from build123d import *

# Parameters (mm, degrees)
SKETCH1_R                    = 3.5
SKETCH1_R_2                  = 1.25
MOUNTING_BOSSES_DEPTH        = 4
MOUNTING_BOSSES_2_DEPTH      = 4
MOUNTING_BOSSES_3_DEPTH      = 4
MOUNTING_BOSSES_4_DEPTH      = 4
MATERIAL_BULK_DEPTH          = 33.5
SKETCH5_R                    = 1.25
MOUNT_POINT_CUT_REPEAT_DEPTH = 67
WEIGHT_RELIEF_DEPTH          = 67
FILLET2_R                    = 5
FILLET3_R                    = 10


with BuildPart() as part:
    # Sketch1 → MOUNTING BOSSES (new body)
    with BuildSketch(Plane.XY):
        with Locations((-30, 54.33)):
            Circle(SKETCH1_R)
        with Locations((-30, 54.33)):
            Circle(SKETCH1_R_2, mode=Mode.SUBTRACT)
    extrude(amount=MOUNTING_BOSSES_DEPTH)



with BuildPart() as body_2:
    # Sketch1 → MOUNTING BOSSES 2 (new body)
    with BuildSketch(Plane.XY):
        with Locations((30, 54.33)):
            Circle(SKETCH1_R)
        with Locations((30, 54.33)):
            Circle(SKETCH1_R_2, mode=Mode.SUBTRACT)
    extrude(amount=MOUNTING_BOSSES_2_DEPTH)


with BuildPart() as body_3:
    # Sketch1 → MOUNTING BOSSES 3 (new body)
    with BuildSketch(Plane.XY):
        with Locations((30, -54.33)):
            Circle(SKETCH1_R)
        with Locations((30, -54.33)):
            Circle(SKETCH1_R_2, mode=Mode.SUBTRACT)
    extrude(amount=MOUNTING_BOSSES_3_DEPTH)


with BuildPart() as body_4:
    # Sketch1 → MOUNTING BOSSES 4 (new body)
    with BuildSketch(Plane.XY):
        with Locations((-30, -54.33)):
            Circle(SKETCH1_R)
        with Locations((-30, -54.33)):
            Circle(SKETCH1_R_2, mode=Mode.SUBTRACT)
    extrude(amount=MOUNTING_BOSSES_4_DEPTH)


with BuildPart() as part_1:
    add(part.part)

    add(body_2.part)  # MATERIAL BULK merges body 2

    add(body_3.part)  # MATERIAL BULK merges body 3

    add(body_4.part)  # MATERIAL BULK merges body 4
    # Sketch4 → MATERIAL BULK (add, symmetric)
    with BuildSketch(Plane(origin=(0, 0, 0), x_dir=(0, 0, -1), z_dir=(1, 0, 0))):
        Polygon((-4, 54.33), (-4, 45.522585119), (0.5, 42.388948755), (0.5, -42.388948755), (-4, -45.522585119), (-4, -54.33), (0, -54.33), (0, -48.83), (5.5, -45), (5.5, 45), (0, 48.83), (0, 54.33), align=None)
    extrude(amount=MATERIAL_BULK_DEPTH, both=True)

    # Sketch5 → MOUNT POINT CUT REPEAT (cut)
    with BuildSketch(Plane.XY):
        with Locations((-30, 54.33)):
            Circle(SKETCH5_R)
        with Locations((30, 54.33)):
            Circle(SKETCH5_R)
        with Locations((30, -54.33)):
            Circle(SKETCH5_R)
        with Locations((-30, -54.33)):
            Circle(SKETCH5_R)
    extrude(amount=MOUNT_POINT_CUT_REPEAT_DEPTH, mode=Mode.SUBTRACT)

    # Sketch6 → WEIGHT RELIEF (cut)
    with BuildSketch(Plane.XY):
        with BuildLine():
            Line((-18.5, 30), (18.5, 30))
            ThreePointArc((18.5, 30), (22.035533906, 28.535533906), (23.5, 25))
            Line((23.5, 25), (23.5, 10))
            ThreePointArc((23.5, 10), (22.035533906, 6.464466094), (18.5, 5))
            Line((18.5, 5), (-18.5, 5))
            ThreePointArc((-18.5, 5), (-22.035533906, 6.464466094), (-23.5, 10))
            Line((-23.5, 10), (-23.5, 25))
            ThreePointArc((-23.5, 25), (-22.035533906, 28.535533906), (-18.5, 30))
        make_face()
        with BuildLine():
            Line((-18.5, -5), (18.5, -5))
            ThreePointArc((18.5, -5), (22.035533906, -6.464466094), (23.5, -10))
            Line((23.5, -10), (23.5, -25))
            ThreePointArc((23.5, -25), (22.035533906, -28.535533906), (18.5, -30))
            Line((18.5, -30), (-18.5, -30))
            ThreePointArc((-18.5, -30), (-22.035533906, -28.535533906), (-23.5, -25))
            Line((-23.5, -25), (-23.5, -10))
            ThreePointArc((-23.5, -10), (-22.035533906, -6.464466094), (-18.5, -5))
        make_face()
    extrude(amount=-WEIGHT_RELIEF_DEPTH, mode=Mode.SUBTRACT)

    # Fillet2
    fillet2_edges = [part_1.edges().sort_by_distance(p)[0] for p in [
        (0, 45.522585119, 4),
        (0, 42.388948755, -0.5),
        (0, -42.388948755, -0.5),
        (0, -45.522585119, 4),
        (0, -48.83, 0),
        (0, -45, -5.5),
        (0, 45, -5.5),
        (0, 48.83, 0),
    ]]
    fillet(fillet2_edges, radius=FILLET2_R)

    # Fillet3
    fillet3_edges = [part_1.edges().sort_by_distance(p)[0] for p in [
        (-26.5, 54.33, 2),
        (26.5, 54.33, 2),
        (26.5, -54.33, 2),
        (-26.5, -54.33, 2),
    ]]
    fillet(fillet3_edges, radius=FILLET3_R)


solid = part_1.part
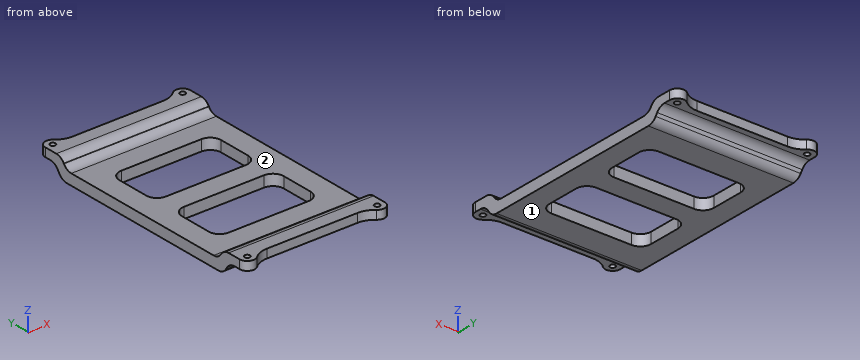
Geometry check sheet. Reference: the model listing, model coordinates, mm. Face numbers are marked on the shaded views. Give positions to 0.01 mm unless a question says otherwise; leave off trailing zeros. Write each loop counter-clockwise with the first axis right and the second up, starting at its lowest first coordinate (ties: lowest second). Pieces come first, ordered by that corner, then holes.
1) Cross-section at C-C (x = 15). Record the boundary of the cut face in (y, z), plus the area to 3 significant figures.
Values follow:
outline: (-54.33, 0) - (-51.44, 0) arc R5 cw to (-47.34, -2.14) - (-46.49, -3.36) arc R5 ccw to (-42.39, -5.5) - (-30, -5.5) - (-30, -0.5) - (-39.78, -0.5) arc R5 cw to (-43.88, 1.64) - (-44.03, 1.86) arc R5 ccw to (-48.13, 4) - (-54.33, 4) - close; (-5, -5.5) - (5, -5.5) - (5, -0.5) - (-5, -0.5) - close; (30, -5.5) - (42.39, -5.5) arc R5 ccw to (46.49, -3.36) - (47.34, -2.14) arc R5 cw to (51.44, 0) - (54.33, 0) - (54.33, 4) - (48.13, 4) arc R5 ccw to (44.03, 1.86) - (43.88, 1.64) arc R5 cw to (39.78, -0.5) - (30, -0.5) - close
area: 305 mm2
2) Cross-section at B-B (x = -30). Record the boundary of the cut face in (y, z), plus the area to 3 significant figures.
Values follow:
outline: (-57.83, 0) - (-55.58, 0) - (-55.58, 4) - (-57.83, 4) - close; (-53.08, 0) - (-51.44, 0) arc R5 cw to (-47.34, -2.14) - (-46.49, -3.36) arc R5 ccw to (-42.39, -5.5) - (42.39, -5.5) arc R5 ccw to (46.49, -3.36) - (47.34, -2.14) arc R5 cw to (51.44, 0) - (53.08, 0) - (53.08, 4) - (48.13, 4) arc R5 ccw to (44.03, 1.86) - (43.88, 1.64) arc R5 cw to (39.78, -0.5) - (-39.78, -0.5) arc R5 cw to (-43.88, 1.64) - (-44.03, 1.86) arc R5 ccw to (-48.13, 4) - (-53.08, 4) - close; (55.58, 0) - (57.83, 0) - (57.83, 4) - (55.58, 4) - close
area: 563 mm2
3) Release check for a two-part mould opening along Y. For the marked faces 1 and 2 record: released by +Y, released by -Y, zero draft, split by the parting line, or undercut.
Values follow:
face 1: zero draft
face 2: undercut
4) Cross-section at A-A (y = -12.5). Record the boundary of the cut face in (x, z).
Values follow:
outline: (-33.5, -5.5) - (-23.5, -5.5) - (-23.5, -0.5) - (-33.5, -0.5) - close; (23.5, -5.5) - (33.5, -5.5) - (33.5, -0.5) - (23.5, -0.5) - close
5) Cross-section at D-D (y = 8.5). Record the boundary of the cut face in (x, z), plus the area to 3 significant figures.
Values follow:
outline: (-33.5, -5.5) - (-23.27, -5.5) - (-23.27, -0.5) - (-33.5, -0.5) - close; (23.27, -5.5) - (33.5, -5.5) - (33.5, -0.5) - (23.27, -0.5) - close
area: 102 mm2
6) Go/stop test with flat-tipped pins: pin 1 Ø2 at (x, z) = (7, 1) entering from +Y; pin 2 Ø4 at (x, z) = (4.5, -3) entering from +Y; pin 3 Ø2 at (x, y) = (30, -54.33) entering from +Z; pin 4 Ø1.2 at (x, z) = (-6.5, 2) entering from -Y. Record where each tip stops, or that it passes through.
Values follow:
pin 1: stops at y = 54.33
pin 2: stops at y = 48.44
pin 3: passes through
pin 4: stops at y = -54.33
7) Thickness scan on line 1 (Y direction, x = -8, z = -4); line 2 (Y direction, x = 8.5, z = -5); line 3 (Y direction, x = -30, z = 2.9). Record the ranges inside material, lowest first.
Values follow:
line 1: y = -45.96 to -30, -5 to 5, 30 to 45.96
line 2: y = -44.57 to -30, -5 to 5, 30 to 44.57
line 3: y = -57.83 to -55.58, -53.08 to -45, 45 to 53.08, 55.58 to 57.83
